Geometry check sheet. Reference: the model listing, model coordinates, mm. A direction names the side the tool comes from. Round coordinates to 2 decimals unless told otherwise and drop trailing zeros. Write each loop counter-clockwise with the first axis right and the second up, starting at its lowest first coordinate (ties: lowest second). Pieces come first, ordered by that corner, then holes. Notation, with made-up numbers: M 72,51.25 L 115,51.25 A15 ccw 115,76.25 Z; hole C 18,-1 d5. An arc over 180 degrees is marked long. Use a Markdown table: item, result.
```python
from build123d import *

# Parameters (mm, degrees)
BOSS_EXTRUDE1_DEPTH = 30
SKETCH4_W           = 30
SKETCH4_H           = 10
CUT_EXTRUDE1_DEPTH  = 22
SKETCH5_W           = 30
SKETCH5_H           = 10
CUT_EXTRUDE2_DEPTH  = 22
SKETCH7_W           = 10
SKETCH7_H           = 30
CUT_EXTRUDE3_DEPTH  = 22


with BuildPart() as part:
    # Sketch1 → Boss-Extrude1 (new body)
    with BuildSketch(Plane.XY):
        Polygon((-52.841994179, 15.40272055), (-12.04436597, -13.503222307), (113.43201935, 7.903510096), (142.337962207, 48.701138306), (139.890104514, 50.435494878), (111.702555671, 10.651802523), (-11.323945253, -10.336970601), (-51.107637608, 17.850578242), align=None)
    extrude(amount=BOSS_EXTRUDE1_DEPTH)

    # Sketch4 → Cut-Extrude1 (cut)
    with BuildSketch(Plane(origin=(1.897901103, -11.124620313, 0), x_dir=(0.9857573554860628, 0.16817382705142964, 0), z_dir=(0.1681738270514296, -0.9857573554860627, 0))):
        with Locations((49.500950021, 10)):
            Rectangle(SKETCH4_W, SKETCH4_H)
    extrude(amount=-CUT_EXTRUDE1_DEPTH, mode=Mode.SUBTRACT)

    # Sketch5 → Cut-Extrude2 (cut)
    with BuildSketch(Plane(origin=(-10.395192144, -14.671695242, 0), x_dir=(0.8159525641948715, -0.5781188571425553, 0), z_dir=(-0.5781188571425553, -0.8159525641948715, 0))):
        with Locations((-27.021163849, 10)):
            Rectangle(SKETCH5_W, SKETCH5_H)
    extrude(amount=-CUT_EXTRUDE2_DEPTH, mode=Mode.SUBTRACT)

    # Sketch7 → Cut-Extrude3 (cut)
    with BuildSketch(Plane(origin=(71.792385036, -50.866353523, 0), x_dir=(0, 0, -1), z_dir=(0.8159525641948736, -0.5781188571425522, 0))):
        with Locations((-10, 97.026078719)):
            Rectangle(SKETCH7_W, SKETCH7_H)
    extrude(amount=-CUT_EXTRUDE3_DEPTH, mode=Mode.SUBTRACT)


solid = part.part
```
Item 1: Go/stop test with flat-tipped pins: pin 1 (6 mm diameter, centred on x = 20, z = 25.5, fed in from +Y); pin 2 (10 mm diameter, centred on x = 55, z = 13, fed in from +Y); pin 3 (10 mm diameter, centred on x = 84.5, z = 19.5, fed in from +Y). Record where each tip stops, or that it passes through.
Outcome:
| item | result |
|---|---|
| pin 1 | stops at y = -4.48 |
| pin 2 | stops at y = 1.76 |
| pin 3 | stops at y = 6.86 |
Item 2: Cross-section at D-D, the plane x = 108.5. Record the cut outline in (y, z), and give its area (3 significant figures).
Outcome:
| item | result |
|---|---|
| outline | M 7.06,0 L 10.11,0 L 10.11,30 L 7.06,30 Z |
| area | 91.3 mm2 |
Item 3: Cross-section at C-C, the plane x = -39. Record the cut outline in (y, z).
Outcome:
| item | result |
|---|---|
| outline | M 5.6,0 L 9.27,0 L 9.27,5 L 5.6,5 Z; M 5.6,15 L 9.27,15 L 9.27,30 L 5.6,30 Z |
Item 4: Material ranges on line 1 along X through (y, z) = (12.5, 6.5); line 2 along Y through (x, z) = (97, 25.75); line 3 along Y through (x, z) = (22, 14.5), recorded low to high. Write a range as from..to.
Outcome:
| item | result |
|---|---|
| line 1 | x = -48.75..-43.56, 113.01..116.69 |
| line 2 | y = 5.1..8.14 |
| line 3 | y = -7.7..-4.65 |
Item 5: Mould release check, pull along X, two halves, no side actions. Record for faces 1 (the face through (52, 0, 30)), 2 (the face through (51.05, 0.304, 18.123)), 3 (the face through (127.683, 28.017, 18.123)): +X half, -X half, draft (parallel to the pull), parting line (faces both ways), or undercut.
Outcome:
| item | result |
|---|---|
| face 1 | draft |
| face 2 | undercut |
| face 3 | +X half |
Item 6: Cross-section at A-A, the plane z = 12. Record the cut outline in (x, y).
Outcome:
| item | result |
|---|---|
| outline | M -52.84,15.4 L -44.68,9.62 L -42.95,12.07 L -51.11,17.85 Z; M -20.2,-7.72 L -12.04,-13.5 L 35.91,-5.32 L 35.4,-2.37 L -11.32,-10.34 L -18.47,-5.27 Z; M 64.98,2.68 L 65.48,-0.28 L 113.43,7.9 L 119.21,16.06 L 116.77,17.8 L 111.7,10.65 Z; M 134.11,42.28 L 136.56,40.54 L 142.34,48.7 L 139.89,50.44 Z |
Item 7: Cross-section at B-B, the plane y = 25.5. Record the cut outline in (x, z), and give its area (3 significant figures).
Outcome:
| item | result |
|---|---|
| outline | M 122.22,0 L 125.9,0 L 125.9,5 L 122.22,5 Z; M 122.22,15 L 125.9,15 L 125.9,30 L 122.22,30 Z |
| area | 73.5 mm2 |
Item 8: Access from +Z, -Z, +X, -X, +Y, -Y to the whole of each face (thin tool, end or side, straight path). Record for faces 4 (the face through (-30.94, 3.56, 18.12)), 5 (the face through (-32.729, 1.152, 18.123)).
Outcome:
| item | result |
|---|---|
| face 4 | +Z, -Z, +Y |
| face 5 | +Z, -Z, -X, -Y |
